```python
from build123d import *

# Parameters (mm, degrees)
SKETCH1_W           = 14
SKETCH1_H           = 30
SKETCH1_R           = 2.1
BOSS_EXTRUDE1_DEPTH = 5.6
CUT_EXTRUDE1_DEPTH  = 4
CHAMFER1_SIZE       = 3
CHAMFER2_SIZE       = 1


with BuildPart() as part:
    # Sketch1 → Boss-Extrude1 (new body)
    with BuildSketch(Plane(origin=(0, 0, 0), x_dir=(1, 0, 0), z_dir=(0, 1, 0))):
        with Locations((7, 15)):
            Rectangle(SKETCH1_W, SKETCH1_H)
        with Locations(Location((7, 22, 0), (0, 0, 270))):
            Circle(SKETCH1_R, mode=Mode.SUBTRACT)
        with Locations(Location((7, 8, 0), (0, 0, 270))):
            Circle(SKETCH1_R, mode=Mode.SUBTRACT)
    extrude(amount=BOSS_EXTRUDE1_DEPTH)

    # Sketch2 → Cut-Extrude1 (cut)
    with BuildSketch(Plane(origin=(0, 5.6, 0), x_dir=(1, 0, 0), z_dir=(0, 1, 0))):
        Polygon((10.55, 24.049593456), (7, 26.099186911), (3.45, 24.049593456), (3.45, 19.950406544), (7, 17.900813089), (10.55, 19.950406544), align=None)
        Polygon((10.55, 10.049593456), (7, 12.099186911), (3.45, 10.049593456), (3.45, 5.950406544), (7, 3.900813089), (10.55, 5.950406544), align=None)
    extrude(amount=-CUT_EXTRUDE1_DEPTH, mode=Mode.SUBTRACT)

    # Chamfer1
    chamfer1_edges = [part.edges().sort_by_distance(p)[0] for p in [
        (0, 2.8, -30),
        (14, 2.8, -30),
        (14, 2.8, 0),
        (0, 2.8, 0),
    ]]
    chamfer(chamfer1_edges, length=CHAMFER1_SIZE)

    # Chamfer2
    chamfer2_edges = [part.edges().sort_by_distance(p)[0] for p in [
        (7, 5.6, -30),
        (14, 5.6, -15),
        (0, 5.6, -15),
        (7, 5.6, 0),
        (12.5, 5.6, -1.5),
        (1.5, 5.6, -1.5),
        (1.5, 5.6, -28.5),
        (12.5, 5.6, -28.5),
    ]]
    chamfer(chamfer2_edges, length=CHAMFER2_SIZE)


solid = part.part
```
Can you work these out from the model? Positions are in its coordinate system, mm. A direction names the side the tool comes from. Coordinates: 2 decimals unless noted, no trailing zeros. Loops run counter-clockwise (first coordinate to the right, second up) from the corner with the lowest first, then second, coordinate; pieces in that order, holes last.
1) Which directions (+Z, -Z, +X, -X, +Y, -Y) give clear straight access to the entire face, cutting with the end or side of a thin tool? Please do faces 4 (the flat face through (13, 2, -28)), 5 (the flat face through (5.2, 3.63, -18.94)).
2) Imagine slicing it at C-C on x = 8. List the corners of the cut face in (y, z) for me, plus the area to 3 significant figures.
3) I need wall thicknesses on probe 1 along Z at (x, y) = (7, 0.7); probe 2 along X at (y, z) = (0.95, -22); probe 3 along Z at (x, y) = (7.5, 4.2). Which ranges of each line are inside material? Lowest first, please.
4) Imagine slicing it at B-B on y = 0.4. List the corners of the cut face in (x, z) for me, plus the area to 3 significant figures.
5) Imagine slicing it at D-D on y = 3.1. List the corners of the cut face in (x, z) for me.
6) Thinking about a two-plate mould opening in X: for faces 1 (the flat face through (7, 5.6, -15)), 2 (the flat face through (14, 2, -15)), 3 (the cylindrical face through (9.082, 0.789, -8.273)), which applies, pulls with the +X half, pulls with the -X half, needs draft (parallel to the pull), parting line crosses it, or undercut?
7) Imagine slicing it at A-A on z = -22. List the corners of the cut face in (x, y) for me.
Completed:
1. face 4: -Z, +X, +Y, -Y
1. face 5: +Y
2. outline: (0, -30) - (4.6, -30) - (5.6, -29) - (5.6, -25.52) - (1.6, -25.52) - (1.6, -23.85) - (0, -23.85) - close; (0, -20.15) - (1.6, -20.15) - (1.6, -18.48) - (5.6, -18.48) - (5.6, -11.52) - (1.6, -11.52) - (1.6, -9.85) - (0, -9.85) - close; (0, -6.15) - (1.6, -6.15) - (1.6, -4.48) - (5.6, -4.48) - (5.6, -1) - (4.6, 0) - (0, 0) - close
2. area: 98.8 mm2
3. probe 1: z = -30 to -24.1, -19.9 to -10.1, -5.9 to 0
3. probe 2: x = 0 to 4.9, 9.1 to 14
3. probe 3: z = -30 to -25.81, -18.19 to -11.81, -4.19 to 0
4. outline: (0, -27) - (3, -30) - (11, -30) - (14, -27) - (14, -3) - (11, 0) - (3, 0) - (0, -3) - close; hole circle Ø4.2 at (7, -22); hole circle Ø4.2 at (7, -8)
4. area: 374 mm2
5. outline: (0, -27) - (3, -30) - (11, -30) - (14, -27) - (14, -3) - (11, 0) - (3, 0) - (0, -3) - close; hole (3.45, -24.05) - (7, -26.1) - (10.55, -24.05) - (10.55, -19.95) - (7, -17.9) - (3.45, -19.95) - close; hole (3.45, -10.05) - (7, -12.1) - (10.55, -10.05) - (10.55, -5.95) - (7, -3.9) - (3.45, -5.95) - close
6. face 1: needs draft
6. face 2: pulls with the +X half
6. face 3: undercut
7. outline: (0, 0) - (4.9, 0) - (4.9, 1.6) - (3.45, 1.6) - (3.45, 5.6) - (1, 5.6) - (0, 4.6) - close; (9.1, 0) - (14, 0) - (14, 4.6) - (13, 5.6) - (10.55, 5.6) - (10.55, 1.6) - (9.1, 1.6) - close
